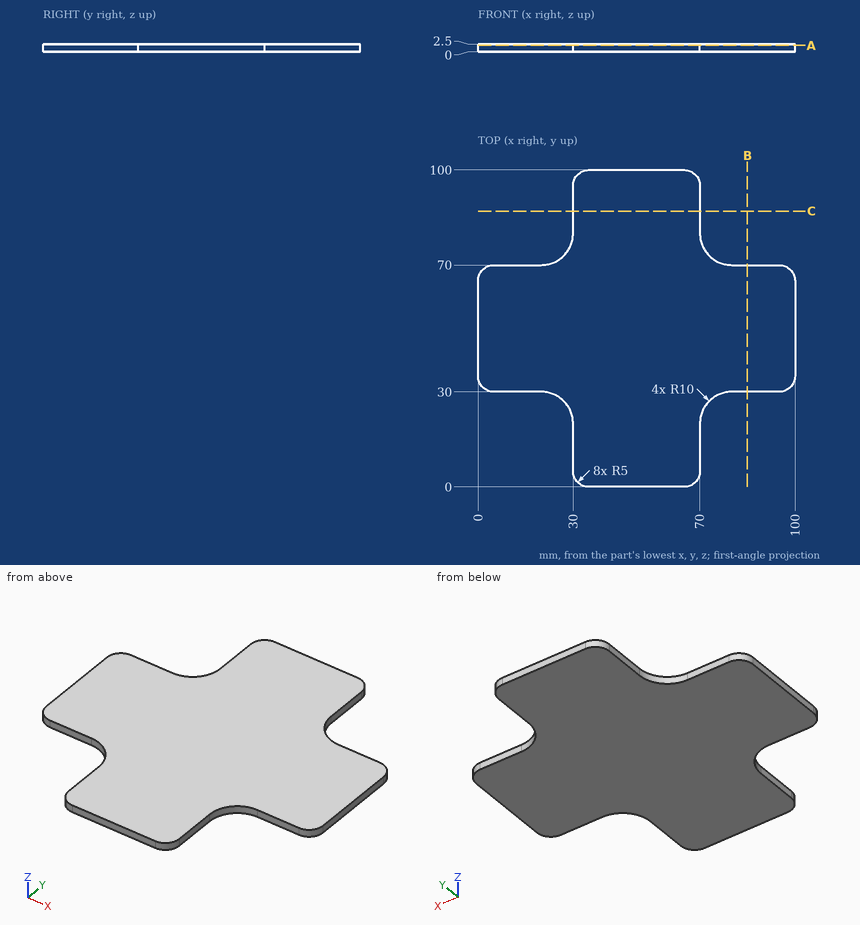
Verification items for this drawing (mm, ordinates from the low corner). Coordinates: 2 decimals unless noted, no trailing zeros. Write each loop counter-clockwise with the first axis right and the second up, starting at its lowest first coordinate (ties: lowest second). Pieces come first, ordered by that corner, then holes. Notation, with made-up numbers: M 51.25,47 L 99.25,47 A20 ccw 99.25,78 Z; hole C 7,14 d4. An arc over 180 degrees is marked long. One line per item, written item: value. Start each with the question number.
(1) Depth check by flat-ended pin: pin 1 (1.2 mm diameter, centred on x = 85.5, z = 1.5, fed in from +Y); pin 2 (0.8 mm diameter, centred on y = 86.5, z = 1.5, fed in from +X); pin 3 (1.2 mm diameter, centred on x = 85, z = 1.5, fed in from -Y). Enter the tip coordinate at first touch or a pass-through.
(2) Sectioned sample at B-B, the plane x = 85. Enter the section's corners in (y, z).
(3) Scan lines: line 1 along X through (y, z) = (80, 1.5); line 2 along Y through (x, z) = (68, 0.45). Record each from-to range of solid material in increasing order. Write a range as [from, to].
(4) Sectioned sample at A-A, the plane z = 2.1. Enter the section's corners in (x, y).
Filled sheet:
1. pin 1: y = 70
1. pin 2: x = 70
1. pin 3: y = 30
2. outline: M 30,0 L 70,0 L 70,2.5 L 30,2.5 Z
3. line 1: [30, 70]
3. line 2: [1, 99]
4. outline: M 0,35 A5 ccw 5,30 L 20,30 A10 cw 30,20 L 30,5 A5 ccw 35,0 L 65,0 A5 ccw 70,5 L 70,20 A10 cw 80,30 L 95,30 A5 ccw 100,35 L 100,65 A5 ccw 95,70 L 80,70 A10 cw 70,80 L 70,95 A5 ccw 65,100 L 35,100 A5 ccw 30,95 L 30,80 A10 cw 20,70 L 5,70 A5 ccw 0,65 Z
